from build123d import *

# Parameters (mm, degrees)
EXTRUDE_1_DEPTH     = 3
SKETCH_2_W          = 3
SKETCH_2_H          = 36.493999941
CUT_EXTRUDE_1_DEPTH = 3
SKETCH_3_W          = 3
SKETCH_3_H          = 3
EXTRUDE_2_DEPTH     = 3


with BuildPart() as part:
    # 스케치1 → 보스-돌출1 (new body)
    with BuildSketch(Plane.XY):
        Polygon((-4.5, 39.543999941), (4.5, 39.543999941), (4.5, -30.443999941), (7, -30.443999941), (7, -39.543999941), (4, -39.543999941), (4, -33.443999941), (-4, -33.443999941), (-4, -39.543999941), (-7, -39.543999941), (-7, -30.443999941), (-4.5, -30.443999941), align=None)
    extrude(amount=EXTRUDE_1_DEPTH)

    # 스케치2 → 컷-돌출1 (cut)
    with BuildSketch(Plane(origin=(0, 0, 0), x_dir=(-1, 0, 0), z_dir=(0, 0, -1))):
        with Locations((0, -15.196999971)):
            Rectangle(SKETCH_2_W, SKETCH_2_H)
    extrude(amount=-CUT_EXTRUDE_1_DEPTH, mode=Mode.SUBTRACT)

    # 스케치3 → 보스-돌출2 (add)
    with BuildSketch(Plane.XY.offset(3)):
        with Locations((-8.5, -35.043999941)):
            Rectangle(SKETCH_3_W, SKETCH_3_H)
        with Locations((8.5, -35.043999941)):
            Rectangle(SKETCH_3_W, SKETCH_3_H)
    extrude(amount=-EXTRUDE_2_DEPTH)


solid = part.part
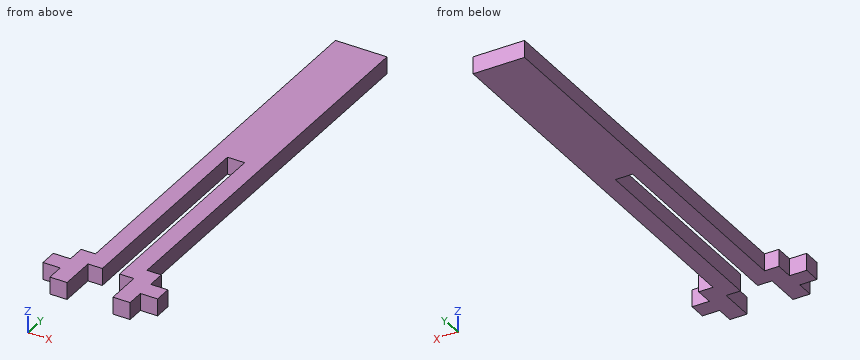
Can you work these out from the model? Positions are in its coordinate system, mm. Round coordinates to 2 decimals unless told otherwise and drop trailing zeros. Order: outer loops, then holes, each group sorted by start corner. A loop starts at its lowest first (then second) coordinate and runs counter-clockwise, first axis right, second up. Notation, with made-up numbers: M 19,35 L 60,35 A23 cw 60,53 Z; hole C 73,-16 d2. An arc over 180 degrees is marked long. Use a Markdown table: item, result.
1) If I drill on line 1 along X through (y, z) = (-27.5, 0.85); line 2 along X through (y, z) = (17.5, 1.4); line 3 along Y through (x, z) = (-3, 2.8), over which ranges is the centre line in solid material (lowest first)?
Geometry says:
| item | result |
|---|---|
| line 1 | x = -4.5 to -1.5, 1.5 to 4.5 |
| line 2 | x = -4.5 to 4.5 |
| line 3 | y = -33.44 to 39.54 |
2) Imagine slicing it at D-D (y = 23.5). List the corners of the cut face in (x, z) for me.
Geometry says:
| item | result |
|---|---|
| outline | M -4.5,0 L 4.5,0 L 4.5,3 L -4.5,3 Z |
3) I'm going to push flat-ended pins straight in: P1, Ø1.5, axis at x = 9, z = 1, coming from the -Y side; P2, Ø1, axis at y = 20, z = 2.5, coming from the +X side; P3, Ø1.5, axis at x = 8.5, z = 2, coming from the +Y side. Where does each tip first touch, or does it pass through?
Geometry says:
| item | result |
|---|---|
| P1 | stops at y = -36.54 |
| P2 | stops at x = 4.5 |
| P3 | stops at y = -33.54 |
4) Imagine slicing it at A-A (y = -26.5). List the corners of the cut face in (x, z) for me.
Geometry says:
| item | result |
|---|---|
| outline | M -4.5,0 L -1.5,0 L -1.5,3 L -4.5,3 Z; M 1.5,0 L 4.5,0 L 4.5,3 L 1.5,3 Z |
5) Imagine slicing it at C-C (x = -6). List the corners of the cut face in (y, z) for me, then the cut area to 3 significant figures.
Geometry says:
| item | result |
|---|---|
| outline | M -39.54,0 L -30.44,0 L -30.44,3 L -39.54,3 Z |
| area | 27.3 mm² |
6) Imagine slicing it at B-B (z = 1.95). List the corners of the cut face in (x, y) for me.
Geometry says:
| item | result |
|---|---|
| outline | M -10,-36.54 L -7,-36.54 L -7,-39.54 L -4,-39.54 L -4,-33.44 L -1.5,-33.44 L -1.5,3.05 L 1.5,3.05 L 1.5,-33.44 L 4,-33.44 L 4,-39.54 L 7,-39.54 L 7,-36.54 L 10,-36.54 L 10,-33.54 L 7,-33.54 L 7,-30.44 L 4.5,-30.44 L 4.5,39.54 L -4.5,39.54 L -4.5,-30.44 L -7,-30.44 L -7,-33.54 L -10,-33.54 Z |
